Answer from the drawing. Dimensions are ordinates in mm from the lowest x, y and z of the part. Round coordinates to 2 decimals unless told otherwise and drop trailing zeros. Loops run counter-clockwise (first coordinate to the right, second up) from the corner with the lowest first, then second, coordinate; pieces in that order, holes last. Notation, with made-up numbers: M -4,24 L 8,24 A33 cw 8,53 Z; hole C 65.25,46 d7. An arc over 180 degrees is marked long. Write each question's results on one line, items separated by ' | '.
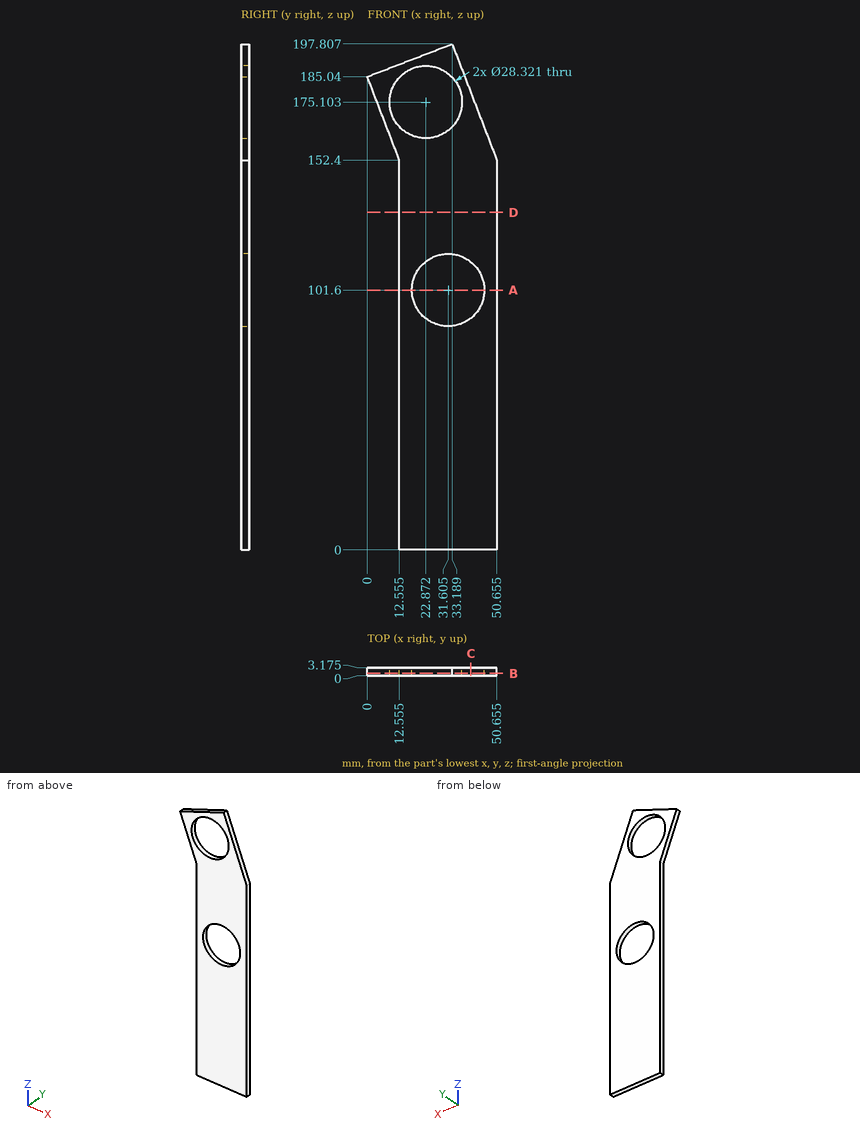
1. Find the intervals of material crossed by L1, parallel to Z at x = 20, y = 0.35 (1 decimal); L2, parallel to Z at x = 29, y = 1.75 (1 decimal); L3, parallel to X at y = 1.6, z = 101.6 (1 decimal), in increasing order.
Completed:
L1: z = 0 to 93.5, 109.7 to 161.2, 189 to 192.7 | L2: z = 0 to 87.7, 115.5 to 162.3, 187.9 to 196.2 | L3: x = 12.6 to 17.4, 45.8 to 50.7
2. Find section D-D, the plane z = 132. Give the vertices of the cut face in (x, y) (1 decimal), then the cut area to 3 significant figures.
Completed:
outline: M 12.6,0 L 50.7,0 L 50.7,3.2 L 12.6,3.2 Z | area: 121 mm2
3. Given P1, Ø1, axis at y = 1, z = 95.5, coming from the -X side (1 decimal), flat-ended and moving along its own axis, determine where the tip first touches the part or whether it passes through.
Completed:
P1: stops at x = 12.6
4. Find section A-A, the plane z = 101.6. Give the vertices of the cut face in (x, y) (1 decimal).
Completed:
outline: M 12.6,0 L 17.4,0 L 17.4,3.2 L 12.6,3.2 Z; M 45.8,0 L 50.7,0 L 50.7,3.2 L 45.8,3.2 Z
5. Find section C-C, the plane x = 40.5. Give the vertices of the cut face in (y, z) (1 decimal).
Completed:
outline: M 0,0 L 3.2,0 L 3.2,90.6 L 0,90.6 Z; M 0,112.6 L 3.2,112.6 L 3.2,178.8 L 0,178.8 Z
6. Find section B-B, the plane y = 1. Give the vertices of the cut face in (x, z) (1 decimal).
Completed:
outline: M 0,185 L 12.6,152.4 L 12.6,0 L 50.7,0 L 50.7,152.4 L 33.2,197.8 Z; hole C 22.9,175.1 d28.3; hole C 31.6,101.6 d28.3
